```python
from build123d import *

# Parameters (mm, degrees)
F0_R     = 3
F1_DEPTH = 36
F2_R     = 6
F3_DEPTH = 2
F4_R     = 0.5
F5_R     = 0.25


with BuildPart() as f1:
    # F0 (on Top) → F1 (new body)
    with BuildSketch(Plane.XY):
        Circle(F0_R)
    extrude(amount=F1_DEPTH)

    # F2 (on face) → F3 (join)
    with BuildSketch(Plane.XY.offset(36)):
        Circle(F2_R)
    extrude(amount=F3_DEPTH)

    # F4
    f4_edges = [f1.edges().sort_by_distance(p)[0] for p in [
        (-6, 0, 38),
    ]]
    fillet(f4_edges, radius=F4_R)

    # F5
    f5_edges = [f1.edges().sort_by_distance(p)[0] for p in [
        (-6, 0, 36),
        (-3, 0, 0),
    ]]
    fillet(f5_edges, radius=F5_R)


solid = f1.part
```
Source: CAD feature listing. Evaluate the final solid. Frame: model axes, mm. A direction names the side the tool comes from. Coordinates: 2 decimals unless noted, no trailing zeros. Write each loop counter-clockwise with the first axis right and the second up, starting at its lowest first coordinate (ties: lowest second). Pieces come first, ordered by that corner, then holes. Notation, with made-up numbers: (20.25, 44) -> (76.25, 44) arc R11 cw to (76.25, 48) -> close; hole circle Ø11 at (45.5, -4). An arc over 180 degrees is marked (long way). Return JSON: item names as keys, results as strings. Group by question number.
1) Ray query, line 1 along Z through (x, y) = (1, -5); line 2 along X through (y, z) = (-1.25, 9.5); line 3 along Y through (x, z) = (1, 13). Return the intervals inside material, ascending.
2) Set-up query: faces 1 (the face through (-3, 0, 18)), 2 (the face through (-6, 0, 37)). Return all of +Z, -Z, +X, -X, +Y, -Y with unobstructed straight access to the full face (end or side cutting, diameter ignored); none if empty.
3) Contact query for flat-ended pins moving along their axis: P1, Ø6, axis at y = -3.5, z = 24.5, coming from the +X side; P2, Ø2, axis at y = -3, z = 19, coming from the +X side; P3, Ø4, axis at x = 2.5, z = 18, coming from the +Y side. Output: stop coordinate, or through.
4) Section query A-A, the plane y = 0. Return loops of the section in (x, z), plus the area to 3 significant figures.
5) Section query C-C, the plane z = 7.5. Return loops of the section in (x, y), plus the area to 3 significant figures.
From the geometry:
{
 "1": {"line 1": "36 to 38", "line 2": "-2.73 to 2.73", "line 3": "-2.83 to 2.83"},
 "2": {"face 1": "-Z", "face 2": "+Z, -Z"},
 "3": {"P1": "x = 2.96", "P2": "x = 2.24", "P3": "y = 2.96"},
 "4": {"outline": "(-6, 36.25) arc R0.25 ccw to (-5.75, 36) -> (-3, 36) -> (-3, 0.25) arc R0.25 ccw to (-2.75, 0) -> (2.75, 0) arc R0.25 ccw to (3, 0.25) -> (3, 36) -> (5.75, 36) arc R0.25 ccw to (6, 36.25) -> (6, 37.5) arc R0.5 ccw to (5.5, 38) -> (-5.5, 38) arc R0.5 ccw to (-6, 37.5) -> close", "area": "240 mm²"},
 "5": {"outline": "circle Ø6 at (0, 0)", "area": "28.3 mm²"}
}
